Design review of the part built by this model. Coordinates are the model's own, in mm. Face numbers are marked on the shaded views. Coordinates: 2 decimals unless noted, no trailing zeros. Loops run counter-clockwise (first coordinate to the right, second up) from the corner with the lowest first, then second, coordinate; pieces in that order, holes last. Notation, with made-up numbers: (66.5, 82.25) - (113.5, 82.25) arc R21 ccw to (113.5, 87.25) - close; hole circle Ø6 at (45.25, 49). An arc over 180 degrees is marked (long way). Return JSON: item names as keys, results as strings. Group by question number.
from build123d import *

# Parameters (mm, degrees)
SKETCH_R        = 19
SKETCH_R_2      = 1.7
PAD_DEPTH       = 3
POCKET_DEPTH    = 50.001
POCKET001_DEPTH = 5
POCKET002_DEPTH = 2.5


with BuildPart() as part:
    # Sketch → Pad (new body)
    with BuildSketch(Plane.XY):
        Polygon((-20, 20), (20, 20), (20, 3), (30, 3), (30, -3), (20, -3), (20, -20), (-20, -20), (-20, -3), (-30, -3), (-30, 3), (-20, 3), align=None)
        Circle(SKETCH_R, mode=Mode.SUBTRACT)
        with Locations((-16, 16)):
            Circle(SKETCH_R_2, mode=Mode.SUBTRACT)
        with Locations((16, 16)):
            Circle(SKETCH_R_2, mode=Mode.SUBTRACT)
        with Locations((-16, -16)):
            Circle(SKETCH_R_2, mode=Mode.SUBTRACT)
        with Locations((16, -16)):
            Circle(SKETCH_R_2, mode=Mode.SUBTRACT)
        with Locations((26, 0)):
            Circle(SKETCH_R_2, mode=Mode.SUBTRACT)
        with Locations((-26, 0)):
            Circle(SKETCH_R_2, mode=Mode.SUBTRACT)
    extrude(amount=PAD_DEPTH)

    # Sketch001 (on Face12 of Pad) → Pocket (cut, through all)
    with BuildSketch(Plane(origin=(-20, 0, 0), x_dir=(0, -1, 0), z_dir=(-1, 0, 0))):
        Polygon((-18, 0), (-20, 2), (-20, 0), align=None)
    extrude(amount=-POCKET_DEPTH, mode=Mode.SUBTRACT)

    # Sketch002 (on Face4 of Pocket) → Pocket001 (cut)
    with BuildSketch(Plane.XY.offset(3)):
        with BuildLine():
            ThreePointArc((-20, -15.999985), (-18.828433, -18.828421), (-16.000001, -20))
            Line((-16.000001, -20), (-16.000001, -25))
            Line((-16.000001, -25), (-25, -25))
            Line((-25, -25), (-25, -15.999985))
            Line((-25, -15.999985), (-20, -15.999985))
        make_face()
        with BuildLine():
            ThreePointArc((16.000017, -20), (18.828428, -18.828426), (20, -16.000015))
            Line((25, -16.000015), (20, -16.000015))
            Line((25, -25), (25, -16.000015))
            Line((16.000017, -25), (25, -25))
            Line((16.000017, -20), (16.000017, -25))
        make_face()
    extrude(amount=-POCKET001_DEPTH, mode=Mode.SUBTRACT)

    # Sketch003 (on Face6 of Pocket001) → Pocket002 (cut)
    with BuildSketch(Plane(origin=(0, 0, 0), x_dir=(1, 0, 0), z_dir=(0, 0, -1))):
        Polygon((14.325, 13.098815), (17.675, 13.098815), (19.35, 16), (17.675, 18.901185), (14.325, 18.901185), (12.65, 16), align=None)
        Polygon((-14.325, 13.098815), (-12.65, 16), (-14.325, 18.901185), (-17.675, 18.901185), (-19.35, 16), (-17.675, 13.098815), align=None)
        Polygon((-14.325, -13.098815), (-17.675, -13.098815), (-19.35, -16), (-17.675, -18.901185), (-14.325, -18.901185), (-12.65, -16), align=None)
        Polygon((14.325, -13.098815), (12.65, -16), (14.325, -18.901185), (17.675, -18.901185), (19.35, -16), (17.675, -13.098815), align=None)
    extrude(amount=-POCKET002_DEPTH, mode=Mode.SUBTRACT)


solid = part.part
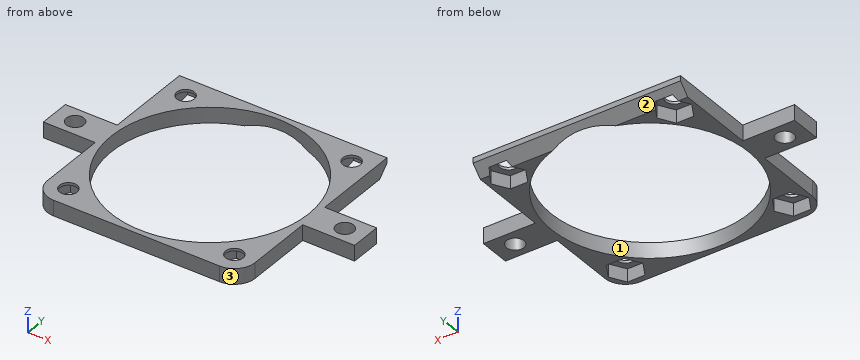
Item 1: Add section A-A (x = 0). State the section outline as (y, z) points, then the cut area to 3 significant figures.
Item 2: Add section B-B (y = -5.5). State the section outline as (x, z) points, then the cut area to 3 significant figures.
Item 3: For P1, Ø2, axis at x = 16, y = -16, coming from the -Z side (3 decimals); P2, Ø1.2, axis at x = 16, z = 1, coming from the +Y side; P3, Ø4.5, axis at x = -16, y = 16, coming from the -Z side; P4, Ø0.9, axis at x = -23.5, z = 1.5, coming from the +Y side, all flat-tipped, find the tip position at first contact; note any pin that passes through.
Item 4: Draft analysis for pull direction X (two halves, no side actions). For the marked faces 1, 2 and 3, state which applies: pulls with the +X half, pulls with the -X half, needs draft (parallel to the pull), parting line crosses it, or undercut.
Item 5: Add section D-D (x = 7.5). State the section outline as (y, z) points, then the cut area to 3 significant figures.
Item 6: To check wall thickness, follow line 1 (X direction, y = -1.5, z = 0.2); line 2 (X direction, y = -16.5, z = 0.25); line 3 (Y direction, x = -16, z = 2.85). State the ranges of each line that lie inside material, in increasing order. Write a range as from..to.
Item 7: Add section C-C (y = 15). State the section outline as (x, z) points.
Answers below:
{
 "1": {"outline": "(-20, 0) - (-19, 0) - (-19, 3) - (-20, 3) - close; (19, 1) - (20, 2) - (20, 3) - (19, 3) - close", "area": "4.50 mm^2"},
 "2": {"outline": "(-20, 0) - (-18.19, 0) - (-18.19, 3) - (-20, 3) - close; (18.19, 0) - (20, 0) - (20, 3) - (18.19, 3) - close", "area": "10.9 mm^2"},
 "3": {"P1": "passes through", "P2": "stops at y = 19.6", "P3": "stops at z = 2.5", "P4": "stops at y = 3"},
 "4": {"face 1": "undercut", "face 2": "needs draft", "face 3": "pulls with the +X half"},
 "5": {"outline": "(-20, 0) - (-17.46, 0) - (-17.46, 3) - (-20, 3) - close; (17.46, 0) - (18, 0) - (20, 2) - (20, 3) - (17.46, 3) - close", "area": "13.3 mm^2"},
 "6": {"line 1": "x = -30..-26.8, -25.2..-18.94, 18.94..25.2, 26.8..30", "line 2": "x = -19.97..-19.06, -12.94..-9.42, 9.42..12.94, 19.06..19.97", "line 3": "y = -20..-17.7, -14.3..-10.25, 10.25..14.3, 17.7..20"},
 "7": {"outline": "(-20, 0) - (-18.77, 0) - (-18.77, 2.5) - (-17.37, 2.5) - (-17.37, 3) - (-20, 3) - close; (-14.63, 2.5) - (-13.23, 2.5) - (-13.23, 0) - (-11.66, 0) - (-11.66, 3) - (-14.63, 3) - close; (11.66, 0) - (13.23, 0) - (13.23, 2.5) - (14.63, 2.5) - (14.63, 3) - (11.66, 3) - close; (17.37, 2.5) - (18.77, 2.5) - (18.77, 0) - (20, 0) - (20, 3) - (17.37, 3) - close"}
}
